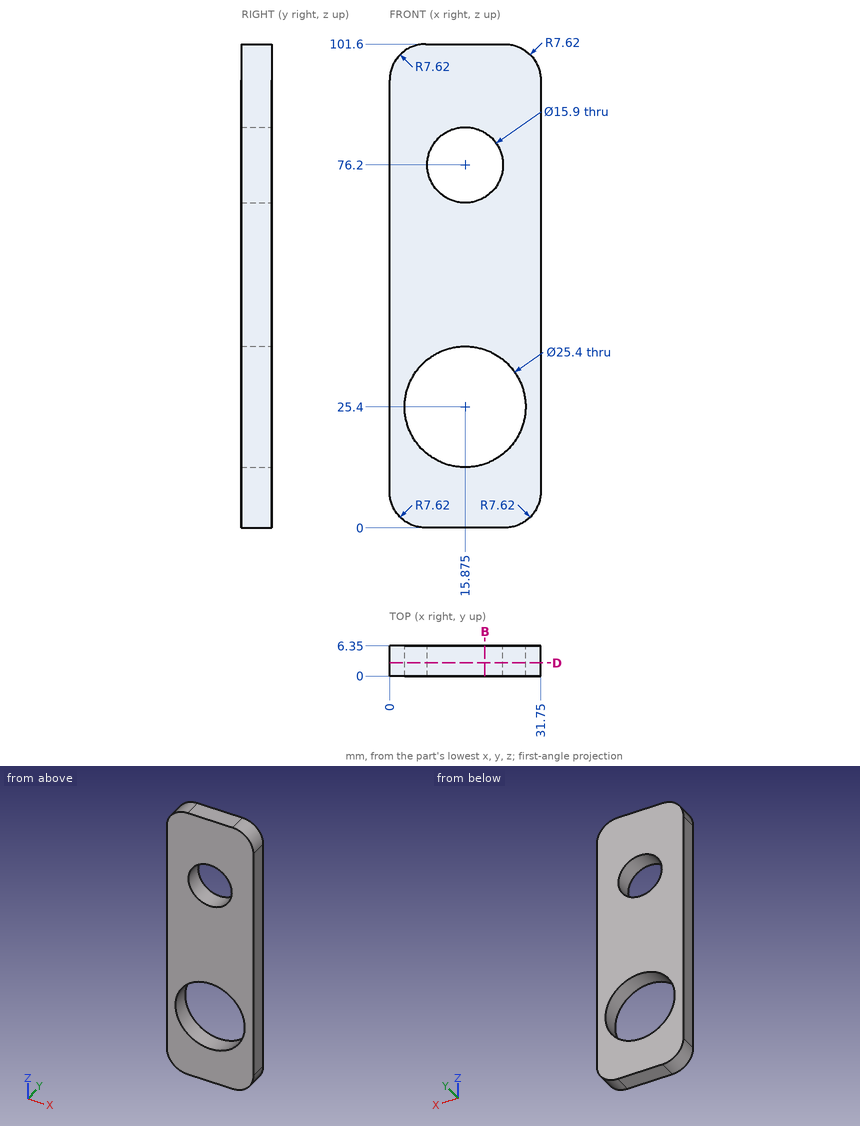
For this review, use the dimensioned drawing (mm, ordinates from the lowest corner) and the shaded views. Round coordinates to 2 decimals unless told otherwise and drop trailing zeros. Write each loop counter-clockwise with the first axis right and the second up, starting at its lowest first coordinate (ties: lowest second). Pieces come first, ordered by that corner, then holes. Notation, with made-up numbers: (63, 78) - (92, 78) arc R6 cw to (92, 86) - close; hole circle Ø7 at (-30, 45.25). An arc over 180 degrees is marked (long way). One line per item, written item: value. Start each with the question number.
1. Consider section D-D on y = 2.75. State how many separate pieces and enclosed holes the cut face has, and give its area (3 significant figures).
2. Clearance check with a flat-ended pin moving along its axis: P1, Ø14.5, axis at x = 15.875, z = 76.2, coming from the +Y side. State where the tip first meets the part, or that it passes through.
3. To check wall thickness, follow L1, parallel to Z at x = 20, y = 4.75 (1 decimal); L2, parallel to Z at x = 23, y = 3.25 (1 decimal); L3, parallel to Z at x = 26, y = 5.5 (1 decimal). State the ranges of each line that lie inside material, in increasing order. Write a range as from..to.
4. Consider section B-B on x = 20. Write out the cut boundary in (y, z), and give its area (3 significant figures).
Checks:
1. separate pieces: 1
1. enclosed holes: 2
1. area: 2,470 mm^2
2. P1: passes through
3. L1: z = 0..13.4, 37.4..69.4, 83..101.6
3. L2: z = 0..14.9, 35.9..72.7, 79.7..101.6
3. L3: z = 0.2..17.7, 33.1..101.4
4. outline: (0, 0) - (6.35, 0) - (6.35, 13.39) - (0, 13.39) - close; (0, 37.41) - (6.35, 37.41) - (6.35, 69.4) - (0, 69.4) - close; (0, 83) - (6.35, 83) - (6.35, 101.6) - (0, 101.6) - close
4. area: 406 mm^2
